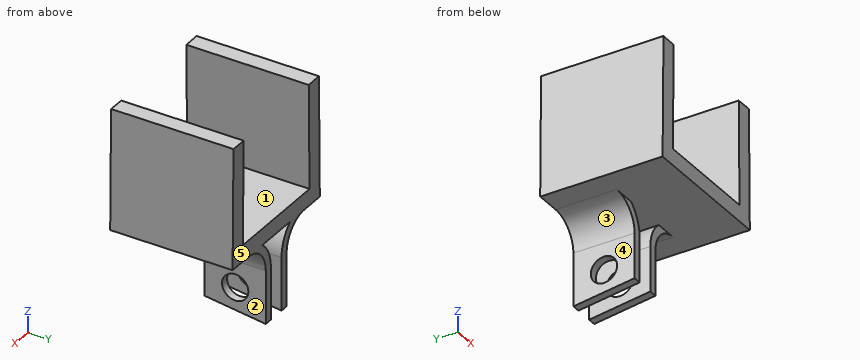
from build123d import *

# Parameters (mm, degrees)
BOSS_EXTRUDE1_DEPTH = 30
BOSS_EXTRUDE2_DEPTH = 15
SKETCH3_R           = 3.225
CUT_EXTRUDE1_DEPTH  = 15
CUT_EXTRUDE3_DEPTH  = 15


with BuildPart() as part:
    # Sketch1 → Boss-Extrude1 (new body)
    with BuildSketch(Plane(origin=(0, 0, 0), x_dir=(1, 0, 0), z_dir=(0, 1, 0))):
        Polygon((-12.8, -12.8), (-13.1, 12.8), (13.1, 12.8), (12.8, -12.6), (16.799721029, -12.6472408), (17.147523085, 16.8), (-17.147149649, 16.8), (-16.79972537, -12.846871782), align=None)
    extrude(amount=BOSS_EXTRUDE1_DEPTH)

    # Sketch2 → Boss-Extrude2 (add)
    with BuildSketch(Plane(origin=(0, 30, 0), x_dir=(1, 0, 0), z_dir=(0, 1, 0))):
        with BuildLine():
            Line((-4.099813282, 36.8), (-4.099813282, 23.785134539))
            ThreePointArc((-4.099813282, 23.785134539), (-6.145711821, 18.845898539), (-11.084947821, 16.8))
            Line((-11.084947821, 16.8), (-5.433351749, 16.8))
            ThreePointArc((-5.433351749, 16.8), (-2.975909846, 19.915231981), (-2.099813282, 23.785134539))
            Line((-2.099813282, 23.785134539), (-2.099813282, 36.8))
            Line((-2.099813282, 36.8), (-4.099813282, 36.8))
        make_face()
        with BuildLine():
            Line((4.100186718, 36.8), (2.100186718, 36.8))
            Line((2.100186718, 36.8), (2.100186718, 23.785134539))
            ThreePointArc((2.100186718, 23.785134539), (2.976283283, 19.915231981), (5.433725186, 16.8))
            Line((5.433725186, 16.8), (11.085321257, 16.8))
            ThreePointArc((11.085321257, 16.8), (6.146085257, 18.845898539), (4.100186718, 23.785134539))
            Line((4.100186718, 23.785134539), (4.100186718, 36.8))
        make_face()
    extrude(amount=-BOSS_EXTRUDE2_DEPTH)

    # Sketch3 → Cut-Extrude1 (cut)
    with BuildSketch(Plane.ZY.offset(4.099813282)):
        with Locations((-30.29256727, 22.5)):
            Circle(SKETCH3_R)
    extrude(amount=-CUT_EXTRUDE1_DEPTH, mode=Mode.SUBTRACT)

    # Sketch8 → Cut-Extrude3 (cut)
    with BuildSketch(Plane(origin=(4.100186718, 0, 0), x_dir=(0, 0, -1), z_dir=(1, 0, 0))):
        Polygon((36.8, 30), (36.8, 15), (34.8, 15), align=None)
    extrude(amount=-CUT_EXTRUDE3_DEPTH, mode=Mode.SUBTRACT)


solid = part.part
Here's how the part is built. I have some questions about the finished solid (model axes, mm). Face numbers are marked on the shaded views. A direction names the side the tool comes from. Round coordinates to 2 decimals unless told otherwise and drop trailing zeros. Order: outer loops, then holes, each group sorted by start corner. A loop starts at its lowest first (then second) coordinate and runs counter-clockwise, first axis right, second up. Notation, with made-up numbers: M 73.25,77 L 86.25,77 A14 cw 86.25,82 Z; hole C 62.5,44.5 d8. An arc over 180 degrees is marked long. Return JSON: item names as keys, results as strings. Group by question number.
1. I'm going to push flat-ended pins straight in: pin 1 Ø4 at (y, z) = (15.5, -14.5) entering from -X; pin 2 Ø6 at (x, y) = (-9.5, 19) entering from -Z; pin 3 Ø7.5 at (y, z) = (22.5, -30.29) entering from -X; pin 4 Ø5 at (y, z) = (22.5, -30.29) entering from -X. Where does each tip first touch, or does it pass through?
2. If we section it at C-C on y = 8.25: List the corners of the cut face in (x, z) for me, then the cut area to 3 significant figures.
3. Please list where these lines run through material, in increasing order: probe 1 along Y at (x, z) = (-4, -30); probe 2 along X at (y, z) = (17.25, -16); probe 3 along X at (y, z) = (26, 5).
4. If we section it at A-A on z = -25: List the corners of the cut face in (x, y) for me.
5. On a 3-axis mill with a long thin cutter (end or side, diameter ignored), from which of +Z, -Z, +X, -X, +Y, -Y can I reach the whole of each face in a straight line? I mean the marked faces 4 and 5. Say none if no direction works.
6. If we section it at B-B on y = 24.5: List the corners of the cut face in (x, z) for me.
7. If we section it at D-D on x = 0: List the corners of the cut face in (y, z) for me.
8. If we mould it in two halves opening along X, with no side actions, what happens to the marked faces 1, 2 and 3? For each: pulls with the +X half, pulls with the -X half, needs draft (parallel to the pull), parting line crosses it, or undercut.
Reply:
{
 "1": {"pin 1": "x = -17.14", "pin 2": "z = -18.52", "pin 3": "x = -4.1", "pin 4": "through"},
 "2": {"outline": "M -17.15,-16.8 L 17.15,-16.8 L 16.8,12.65 L 12.8,12.6 L 13.1,-12.8 L -13.1,-12.8 L -12.8,12.8 L -16.8,12.85 Z", "area": "341 mm^2"},
 "3": {"probe 1": "15 to 19.29, 25.71 to 30", "probe 2": "-17.14 to 17.14", "probe 3": "-16.89 to -12.89, 12.89 to 16.89"},
 "4": {"outline": "M -4.1,15 L -2.1,15 L -2.1,30 L -4.1,30 Z; M 2.1,15 L 4.1,15 L 4.1,30 L 2.1,30 Z"},
 "5": {"face 4": "-Z, -X, +Y, -Y", "face 5": "+Z, -Z, +X, -X, +Y"},
 "6": {"outline": "M -17.15,-16.8 L -11.08,-16.8 A6.99 cw -4.1,-23.79 L -4.1,-27.76 L -2.1,-27.76 L -2.1,-23.79 A8.99 ccw -5.43,-16.8 L 5.43,-16.8 A8.99 ccw 2.1,-23.79 L 2.1,-27.76 L 4.1,-27.76 L 4.1,-23.79 A6.99 cw 11.09,-16.8 L 17.15,-16.8 L 16.8,12.65 L 12.8,12.6 L 13.1,-12.8 L -13.1,-12.8 L -12.8,12.8 L -16.8,12.85 Z; M -4.1,-36.07 L -2.1,-36.07 L -2.1,-32.82 L -4.1,-32.82 Z; M 2.1,-36.07 L 4.1,-36.07 L 4.1,-32.82 L 2.1,-32.82 Z"},
 "7": {"outline": "M 0,-16.8 L 30,-16.8 L 30,-12.8 L 0,-12.8 Z"},
 "8": {"face 1": "undercut", "face 2": "pulls with the +X half", "face 3": "pulls with the -X half"}
}
